Part model, mm, in its own coordinate system. Face numbers are marked on the shaded views. A direction names the side the tool comes from. Round coordinates to 2 decimals unless told otherwise and drop trailing zeros. Write each loop counter-clockwise with the first axis right and the second up, starting at its lowest first coordinate (ties: lowest second). Pieces come first, ordered by that corner, then holes. Notation, with made-up numbers: M 59,13.5 L 77,13.5 A26 ccw 77,36.5 Z; hole C 1,67 d3. An arc over 180 degrees is marked long. Use a Markdown table: item, result. Add a question column.
1) Wall check: probe 1 along Z at (x, y) = (0, -2.6) (3 decimals); probe 2 along Y at (x, z) = (-5, 17); probe 3 along Z at (x, y) = (2.5, -5.5). Give the ranges that are in metal, low to high.
2) Slice it at A-A on y = -2.25. Write the cut outline in (x, z) (3 decimals).
3) Two-plate mould, pull along X, no slides. Class the marked faces 1, 2 and 3: released by +X, released by -X, zero draft, split by the parting line, or undercut.
4) Slice it at D-D on z = 17. Write the cut outline in (x, y), plus the area to 3 significant figures.
5) Which spindle directions (+Z, -Z, +X, -X, +Y, -Y) get a long thin tool onto all of the face, cutting with end or side? Do the marked faces 4, 5 and 6. Say none if no direction does.
6) Drop flat-ended pins along their axis: P1, Ø2, axis at x = -1, z = 15.5, coming from the +Y side; P2, Ø6, axis at x = -7, y = -9, coming from the -Z side; P3, Ø10.5, axis at x = 0, z = 0, coming from the -Y side; P4, Ø7, axis at x = 1.5, z = 12, coming from the -Y side. Give the stop position or say it passes through.
7) Slice it at C-C on z = 0. Write the cut outline in (x, y) (3 decimals).
8) Slice it at B-B on x = 0. Write the cut outline in (y, z) (3 decimals).
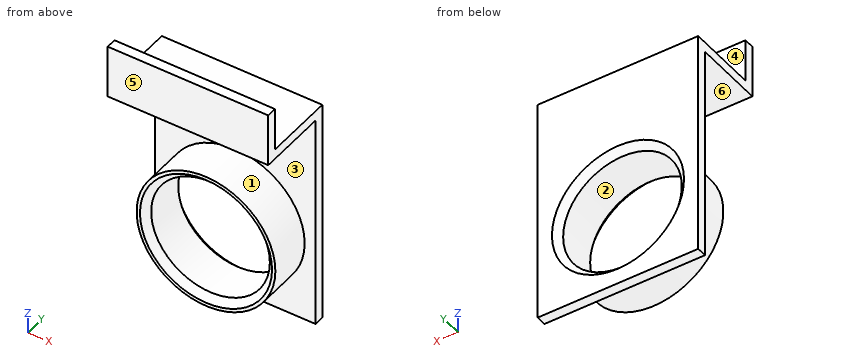
```python
from build123d import *

# Parameters (mm, degrees)
F1_W          = 1.5
F1_H          = 6.5
F1_H_2        = 1.5
F2_DEPTH      = 12
F2_DEPTH_BACK = 12
F0_R          = 8.875
F3_DEPTH      = 25
F0_R_2        = 10.375
F4_DEPTH      = 8
F5_SIZE       = 1


with BuildPart() as f2:
    # F1 (on Right) → F2 (new body, two sides)
    with BuildSketch(Plane.YZ) as f2_sk:
        Polygon((-1.5, -12.204361), (0, -12.204361), (0, 20.509552), (0, 22.009552), (-1.5, 22.009552), (-10.5, 22.009552), (-10.5, 20.509552), (-1.5, 20.509552), align=None)
        with Locations((-11.25, 25.259552)):
            Rectangle(F1_W, F1_H)
        with Locations((-11.25, 21.259552)):
            Rectangle(F1_W, F1_H_2)
    extrude(amount=F2_DEPTH)
    extrude(f2_sk.sketch, amount=-F2_DEPTH_BACK)

    # F0 (on Front) → F3 (cut)
    with BuildSketch(Plane.XZ):
        Circle(F0_R)
    extrude(amount=F3_DEPTH, mode=Mode.SUBTRACT)

    # F0 (on Front) → F4 (join)
    with BuildSketch(Plane.XZ):
        Circle(F0_R_2)
        Circle(F0_R, mode=Mode.SUBTRACT)
    extrude(amount=F4_DEPTH)

    # F5
    f5_edges = [f2.edges().sort_by_distance(p)[0] for p in [
        (-8.875, -8, 0),
        (-8.875, 0, 0),
    ]]
    chamfer(f5_edges, length=F5_SIZE)


solid = f2.part
```
Entries:
| question | item | result |
|---|---|---|
| 1 | probe 1 | z = -10.375 to -8.875, 8.875 to 10.375, 20.51 to 22.01 |
| 1 | probe 2 | y = -1.5 to 0 |
| 1 | probe 3 | z = -10.07 to -8.52, 8.52 to 10.07, 20.51 to 22.01 |
| 2 | outline | M -12,20.51 L 12,20.51 L 12,22.01 L -12,22.01 Z; C 0,0 d20.75; hole C 0,0 d17.75 |
| 3 | face 1 | split by the parting line |
| 3 | face 2 | undercut |
| 3 | face 3 | zero draft |
| 4 | outline | M -12,-1.5 L 12,-1.5 L 12,0 L -12,0 Z |
| 4 | area | 36.0 mm^2 |
| 5 | face 4 | +Z, +X, -X, +Y |
| 5 | face 5 | +Z, -Z, +X, -X, -Y |
| 5 | face 6 | +X, -X, -Y |
| 6 | P1 | stops at y = 0 |
| 6 | P2 | stops at z = -9.5 |
| 6 | P3 | passes through |
| 6 | P4 | stops at y = -8 |
| 7 | outline | M -12,-1.5 L -10.375,-1.5 L -10.375,-8 L -9.875,-8 L -8.875,-7 L -8.875,-1 L -9.875,0 L -12,0 Z; M 8.875,-7 L 9.875,-8 L 10.375,-8 L 10.375,-1.5 L 12,-1.5 L 12,0 L 9.875,0 L 8.875,-1 Z |
| 8 | outline | M -12,20.51 L -1.5,20.51 L -1.5,10.375 L -8,10.375 L -8,9.875 L -7,8.875 L -1,8.875 L 0,9.875 L 0,22.01 L -10.5,22.01 L -10.5,28.51 L -12,28.51 Z; M -8,-10.375 L -1.5,-10.375 L -1.5,-12.204 L 0,-12.204 L 0,-9.875 L -1,-8.875 L -7,-8.875 L -8,-9.875 Z |
